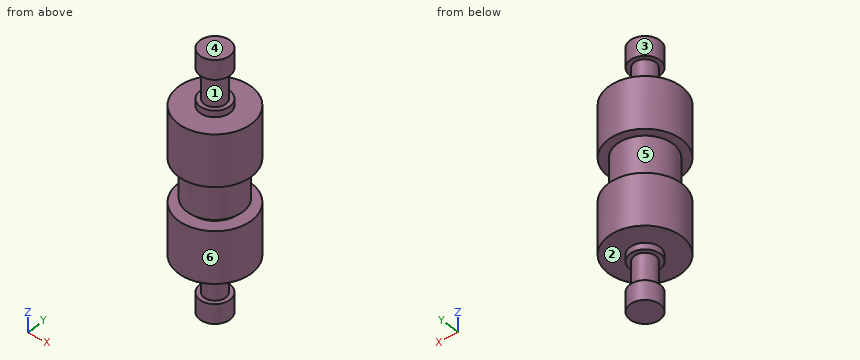
Autodesk Fusion 360 part; units mm, degrees
sketch "Sketch1" plane through (0, 0, 0) normal (0, 0, 1) x (1, 0, 0)
  circle A0 centre (0, 0) radius 3.5
  circle A1 centre (0, 0) radius 8.5
  circle A2 centre (0, 0) radius 2.5
  circle A3 centre (0, 0) radius 6.5
  circle A4 centre (0, 0) radius 5.5
  dimension "d1" = 7
  dimension "d2" = 5
  dimension "d10" = -1
  dimension "d17" = -2
  dimension "d21" = -1
extrude "Extrude1" add sketch "Sketch1" along normal blind 60 contours A0 | A1 | A2 | A3 | A4
extrude "Extrude2" cut sketch "Sketch1" along normal blind 13 contours A1 | A3 | A4
extrude "Extrude3" cut sketch "Sketch1" against normal blind 13 from surface at 60 contours A1 | A3 | A4
extrude "Extrude4" cut sketch "Sketch1" along normal blind 7 from surface at 4.5 contours A0
extrude "Extrude5" cut sketch "Sketch1" against normal blind 7 from surface at 55.5 contours A0
extrude "Extrude6" cut sketch "Sketch1" along normal blind 10 from surface at 25 contours A1
extrude "Extrude7" cut sketch "Sketch1" along normal blind 1 from surface at 25 contours A3
extrude "Extrude8" cut sketch "Sketch1" along normal blind 1 from surface at 25 contours A3
extrude "Extrude9" cut sketch "Sketch1" along normal blind 1 from surface at 25 contours A3
extrude "Extrude10" cut sketch "Sketch1" along normal blind 1 from surface at 25 contours A3
extrude "Extrude11" cut sketch "Sketch1" along normal blind 1 from surface at 25 contours A3
Could you check a few things on this model? Use its own coordinates, in mm. Face numbers are marked on the shaded views. A direction names the side the tool comes from. Round coordinates to 2 decimals unless told otherwise and drop trailing zeros. Write each loop counter-clockwise with the first axis right and the second up, starting at its lowest first coordinate (ties: lowest second). Pieces come first, ordered by that corner, then holes. Notation, with made-up numbers: (22.25, 80) - (32.25, 80) arc R29 cw to (32.25, 111) - close; hole circle Ø1 at (38.25, -12). An arc over 180 degrees is marked (long way). Put each result on its own line as item: value. Start each with the question number.
(1) I want a section at B-B, the plane z = 42. Please give me the cut outline in (x, y).
(2) Thinking about a two-plate mould opening in Z: for the marked faces 4, 5 and 6, which applies, released by +Z, released by -Z, zero draft, split by the parting line, or undercut?
(3) For the marked faces 1, 2 and 3, which set-ups out of +Z, -Z, +X, -X, +Y, -Y let a thin tool reach every point of the face, with its end or its side?
(4) I want a section at A-A, the plane z = 54. Please give me the cut outline in (x, y).
(5) Will these pins go through, and if not, where does the flat tip stop? pin 1 (5 mm diameter, centred on y = 0.5, z = 28.5, fed in from -X); pin 2 (8.5 mm diameter, centred on x = -3.5, y = -1.5, fed in from -Z); pin 3 (3 mm diameter, centred on x = -4.5, z = 46.5, fed in from +Y); pin 4 (6 mm diameter, centred on x = -6.5, z = 53, fed in from +Y).
(6) I need wall thicknesses on probe 1 along Z at (x, y) = (1.75, -3); probe 2 along Z at (x, y) = (0.75, 8.25); probe 3 along Z at (x, y) = (-2, 5). Which ranges of each line are inside material? Lowest first, please.
Here are the results:
1. outline: circle Ø17 at (0, 0)
2. face 4: released by +Z
2. face 5: undercut
2. face 6: zero draft
3. face 1: none
3. face 2: -Z
3. face 3: +Z
4. outline: circle Ø5 at (0, 0)
5. pin 1: stops at x = -6.5
5. pin 2: stops at z = 0
5. pin 3: stops at y = 7.95
5. pin 4: passes through
6. probe 1: z = 0 to 4.5, 11.5 to 48.5, 55.5 to 60
6. probe 2: z = 13 to 25, 35 to 47
6. probe 3: z = 13 to 47
